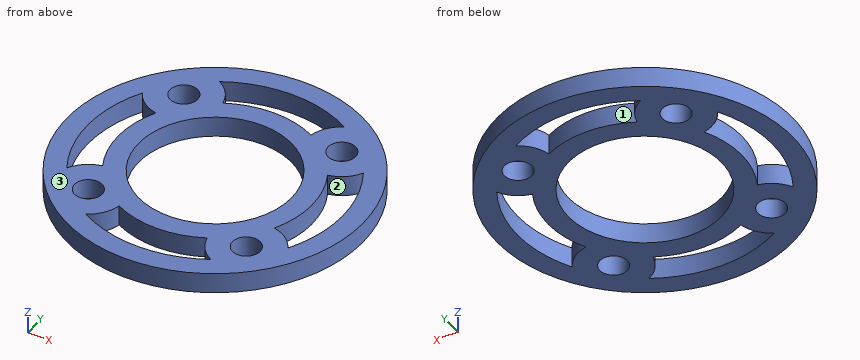
from build123d import *

# Parameters (mm, degrees)
F0_R            = 23.01875
F0_R_2          = 2.15265
F0_R_3          = 11.90625
F1_DEPTH        = 3.175
F3_DEPTH        = 3.175
F3_COPIES_COUNT = 4


# Not quite as in the source:
# - a pattern or mirror of a feature is missing from the dataset's text; its kind, count and spacing are read off the source's solid


with BuildPart() as f1:
    # F0 (on Top) → F1 (new body)
    with BuildSketch(Plane.XY):
        Circle(F0_R)
        with Locations((-12.3478521665, -12.3478521665)):
            Circle(F0_R_2, mode=Mode.SUBTRACT)
        with Locations((12.3478521665, -12.3478521665)):
            Circle(F0_R_2, mode=Mode.SUBTRACT)
        with Locations((-12.3478521665, 12.3478521665)):
            Circle(F0_R_2, mode=Mode.SUBTRACT)
        Circle(F0_R_3, mode=Mode.SUBTRACT)
        with Locations((12.3478521665, 12.3478521665)):
            Circle(F0_R_2, mode=Mode.SUBTRACT)
    extrude(amount=F1_DEPTH)

    # F2 (on face) → F3 (cut, through all)
    with BuildSketch(Plane.XY.offset(3.175)):
        with BuildLine():
            ThreePointArc((-9.7719120136, 17.2709047146), (-7.8938999882, 15.6696324205), (-6.8946489019, 13.4129757356))
            ThreePointArc((-6.8946489019, 13.4129757356), (0, 15.08125), (6.8946489019, 13.4129757356))
            ThreePointArc((6.8946489019, 13.4129757356), (7.8938999882, 15.6696324205), (9.7719120136, 17.2709047146))
            ThreePointArc((9.7719120136, 17.2709047146), (0, 19.84375), (-9.7719120136, 17.2709047146))
        make_face()
    f3 = extrude(amount=-F3_DEPTH, mode=Mode.SUBTRACT)

    # F3_copies: F3 ×4 about axis
    f3_copies_axis = Axis((0, 0, 0), (0, 0, 1))
    for i in range(1, F3_COPIES_COUNT):
        add(f3.rotate(f3_copies_axis, i * 360 / F3_COPIES_COUNT), mode=Mode.SUBTRACT)


solid = f1.part
For this review, take the finished solid that the model builds, in its own axes (mm). Face numbers are marked on the shaded views. Round coordinates to 2 decimals unless told otherwise and drop trailing zeros. Loops run counter-clockwise (first coordinate to the right, second up) from the corner with the lowest first, then second, coordinate; pieces in that order, holes last. Notation, with made-up numbers: (-7.75, -33) - (13.25, -33) arc R22 cw to (13.25, 5) - close; hole circle Ø8 at (25.5, 47). An arc over 180 degrees is marked (long way). Answer as CSV lines item,"result".
(1) Consider section C-C on z = 1.55. Give the number of separate pieces and of enclosed holes in the cut face, then the cut area to 3 significant figures.
Checked values:
separate pieces,"1"
enclosed holes,"9"
area,"844 mm2"
(2) Wall thickness on line 1 (Y direction, x = -5.5, z = 0.9); line 2 (X direction, y = 1, z = 2.7); line 3 (Y direction, x = 10.5, z = 0.2): over which ranges is each line inside the solid? List them lowest first.
Checked values:
line 1,"y = -22.35 to -19.07, -14.04 to -10.56, 10.56 to 14.04, 19.07 to 22.35"
line 2,"x = -23 to -19.82, -15.05 to -11.86, 11.86 to 15.05, 19.82 to 23"
line 3,"y = -20.48 to -13.45, -11.24 to -5.61, 5.61 to 11.24, 13.45 to 20.48"
(3) Mouldability with a two-part tool opening along X and no side actions: class the marked faces 1, 2 and 3 as +X half, -X half, draft (parallel to the pull), parting line (faces both ways), or undercut.
Checked values:
face 1,"undercut"
face 2,"undercut"
face 3,"draft"
(4) Insertion check: P1, Ø7, axis at x = -12.35, y = 12.35, coming from the +Z side (3 decimals); P2, Ø1, axis at y = -7.5, z = 2, coming from the +X side. Each pin has a flat end and moves straight along its axis. Give the tip position at first contact, or say it passes through.
Checked values:
P1,"stops at z = 3.175"
P2,"stops at x = 21.93"
(5) Consider section A-A on y = 0. Give the boundary of the cut face in (x, z) (3 decimals).
Checked values:
outline,"(-23.019, 0) - (-19.844, 0) - (-19.844, 3.175) - (-23.019, 3.175) - close; (-15.081, 0) - (-11.906, 0) - (-11.906, 3.175) - (-15.081, 3.175) - close; (11.906, 0) - (15.081, 0) - (15.081, 3.175) - (11.906, 3.175) - close; (19.844, 0) - (23.019, 0) - (23.019, 3.175) - (19.844, 3.175) - close"
